Check sheet for the modelled part. Datum: model origin and axes. Units: mm. Coordinates: 2 decimals unless noted, no trailing zeros. Loops run counter-clockwise (first coordinate to the right, second up) from the corner with the lowest first, then second, coordinate; pieces in that order, holes last. Notation, with made-up numbers: (-10.5, 3) - (4.5, 3) arc R20 ccw to (4.5, 32) - close; hole circle Ø2 at (14, 36.25). An arc over 180 degrees is marked (long way). Write each question's results on one line, items separated by ' | '. Start each with the question number.
1. Cross-section at A-A (z = 30). Record the cut outline in (x, y), and give its area (3 significant figures).
2. Cross-section at D-D (x = 47.5). Record the cut outline in (y, z).
3. Thickness scan on line 1 (X direction, y = 41.7, z = 20); line 2 (X direction, y = 41, z = -21); line 3 (X direction, y = 40.75, z = 10). Record the ranges inside material, lowest first. Write a range as [from, to].
4. Cross-section at C-C (x = 27.5). Record the cut outline in (y, z), and give its area (3 significant figures).
5. Gauge pin test, flat ends, axial feed: P1, Ø1.5, axis at y = 41, z = -36, coming from the -X side; P2, Ø1.5, axis at y = 42, z = -11.5, coming from the +X side; P3, Ø1.5, axis at y = 41.5, z = 3.5, coming from the -X side. Record the tip position at first contact, or that the pin passes through.
6. Cross-section at B-B (z = -11). Record the cut outline in (x, y).
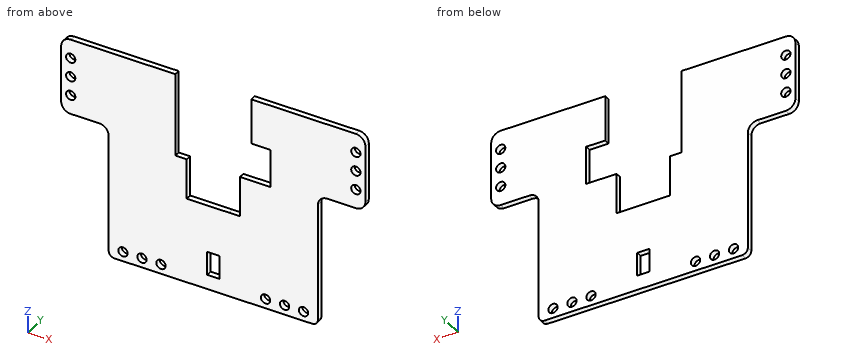
```python
from build123d import *

# Parameters (mm, degrees)
SKETCH2_W           = 6.4
SKETCH2_H           = 12.35
SKETCH2_R           = 2.45
BOSS_EXTRUDE1_DEPTH = 3


with BuildPart() as part:
    # Sketch2 → Boss-Extrude1 (new body)
    with BuildSketch(Plane(origin=(0, 40, 0), x_dir=(1, 0, 0), z_dir=(0, 1, 0))):
        with BuildLine():
            Line((30, -16.164928148), (20, -16.164928148))
            Line((20, -16.164928148), (20, -40))
            Line((20, -40), (75, -40))
            ThreePointArc((75, -40), (78.535533906, -38.535533906), (80, -35))
            Line((80, -35), (80, -5))
            ThreePointArc((80, -5), (78.535533906, -1.464466094), (75, 0))
            Line((75, 0), (60, 0))
            ThreePointArc((60, 0), (56.464466094, 1.464466094), (55, 5))
            Line((55, 5), (55, 67))
            ThreePointArc((55, 67), (54.121320344, 69.121320344), (52, 70))
            Line((52, 70), (-52, 70))
            ThreePointArc((-52, 70), (-54.121320344, 69.121320344), (-55, 67))
            Line((-55, 67), (-55, 5))
            ThreePointArc((-55, 5), (-56.464466094, 1.464466094), (-60, 0))
            Line((-60, 0), (-75, 0))
            ThreePointArc((-75, 0), (-78.535533906, -1.464466094), (-80, -5))
            Line((-80, -5), (-80, -35))
            ThreePointArc((-80, -35), (-78.535533906, -38.535533906), (-75, -40))
            Line((-75, -40), (-20, -40))
            Line((-20, -40), (-20, 3.835071852))
            Line((-20, 3.835071852), (-14, 3.835071852))
            Line((-14, 3.835071852), (-14, 25))
            Line((-14, 25), (8.289849185, 25))
            Line((8.289849185, 25), (14, 25.022996562))
            Line((14, 25.022996562), (14, 3.835071852))
            Line((14, 3.835071852), (30, 3.835071852))
            Line((30, 3.835071852), (30, -16.164928148))
        make_face()
        with Locations((0, 56.175)):
            Rectangle(SKETCH2_W, SKETCH2_H, mode=Mode.SUBTRACT)
        with Locations(Location((-75, -30, 0), (0, 0, 270))):
            Circle(SKETCH2_R, mode=Mode.SUBTRACT)
        with Locations(Location((-75, -20, 0), (0, 0, 270))):
            Circle(SKETCH2_R, mode=Mode.SUBTRACT)
        with Locations(Location((-75, -10, 0), (0, 0, 270))):
            Circle(SKETCH2_R, mode=Mode.SUBTRACT)
        with Locations(Location((75, -30, 0), (0, 0, 270))):
            Circle(SKETCH2_R, mode=Mode.SUBTRACT)
        with Locations(Location((75, -20, 0), (0, 0, 270))):
            Circle(SKETCH2_R, mode=Mode.SUBTRACT)
        with Locations(Location((75, -10, 0), (0, 0, 270))):
            Circle(SKETCH2_R, mode=Mode.SUBTRACT)
        with Locations(Location((-47.5, 65, 0), (0, 0, 270))):
            Circle(SKETCH2_R, mode=Mode.SUBTRACT)
        with Locations(Location((-37.5, 65, 0), (0, 0, 270))):
            Circle(SKETCH2_R, mode=Mode.SUBTRACT)
        with Locations(Location((-27.5, 65, 0), (0, 0, 270))):
            Circle(SKETCH2_R, mode=Mode.SUBTRACT)
        with Locations(Location((27.5, 65, 0), (0, 0, 270))):
            Circle(SKETCH2_R, mode=Mode.SUBTRACT)
        with Locations(Location((37.5, 65, 0), (0, 0, 270))):
            Circle(SKETCH2_R, mode=Mode.SUBTRACT)
        with Locations(Location((47.5, 65, 0), (0, 0, 270))):
            Circle(SKETCH2_R, mode=Mode.SUBTRACT)
    extrude(amount=BOSS_EXTRUDE1_DEPTH)


solid = part.part
```
Established:
1) outline: (-80, 40) - (-77.45, 40) - (-77.45, 43) - (-80, 43) - close; (-72.55, 40) - (-20, 40) - (-20, 43) - (-72.55, 43) - close; (20, 40) - (72.55, 40) - (72.55, 43) - (20, 43) - close; (77.45, 40) - (80, 40) - (80, 43) - (77.45, 43) - close | area: 331 mm^2
2) outline: (40, -70) - (43, -70) - (43, -67.45) - (40, -67.45) - close; (40, -62.55) - (43, -62.55) - (43, 40) - (40, 40) - close
3) line 1: [-80, -77.45], [-72.55, -20], [20, 72.55], [77.45, 80] | line 2: [-55, -14], [14, 55] | line 3: [-80, -77.45], [-72.55, -20], [30, 72.55], [77.45, 80]
4) outline: (40, -70) - (43, -70) - (43, -67.45) - (40, -67.45) - close; (40, -62.55) - (43, -62.55) - (43, -3.84) - (40, -3.84) - close; (40, 16.16) - (43, 16.16) - (43, 40) - (40, 40) - close | area: 255 mm^2
5) P1: x = -55 | P2: x = 55 | P3: x = -79.94
6) outline: (-55, 40) - (-14, 40) - (-14, 43) - (-55, 43) - close; (14, 40) - (55, 40) - (55, 43) - (14, 43) - close
